Geometry: final body of the model. Coordinates: model frame, mm. A direction names the side the tool comes from. Round coordinates to 2 decimals unless told otherwise and drop trailing zeros. Loops run counter-clockwise (first coordinate to the right, second up) from the corner with the lowest first, then second, coordinate; pieces in that order, holes last. Notation, with made-up numbers: M 86,-30 L 139,-30 A9 cw 139,-18 Z; hole C 62,-4 d10. An arc over 180 degrees is marked long. Write each question's results on one line, items separated by ' | '.
```python
from build123d import *

# Parameters (mm, degrees)
BOSS_EXTRUDE1_DEPTH = 80
SKETCH2_W           = 20
SKETCH2_H           = 28
BOSS_EXTRUDE2_DEPTH = 10
FILLET1_R           = 7
CUT_EXTRUDE1_DEPTH  = 20
FILLET2_R           = 7
SKETCH4_R           = 3.2
CUT_EXTRUDE2_DEPTH  = 9.5


with BuildPart() as part:
    # Sketch1 → Boss-Extrude1 (new body)
    with BuildSketch(Plane.XY):
        Polygon((0, 0), (0, 34.685337878), (60.076767483, 0), align=None)
    extrude(amount=BOSS_EXTRUDE1_DEPTH)

    # Sketch2 → Boss-Extrude2 (add)
    with BuildSketch(Plane.XY.offset(80)):
        with Locations((10, -4)):
            Rectangle(SKETCH2_W, SKETCH2_H)
    boss_extrude2 = extrude(amount=BOSS_EXTRUDE2_DEPTH)

    # Fillet1
    fillet1_edges = [part.edges().sort_by_distance(p)[0] for p in [
        (20, 5, 80),
        (10, 10, 80),
    ]]
    fillet(fillet1_edges, radius=FILLET1_R)

    # Sketch3 → Cut-Extrude1 (cut)
    with BuildSketch(Plane.XY.offset(90)):
        with BuildLine():
            Line((7, -12), (7, -8))
            ThreePointArc((7, -8), (10, -5), (13, -8))
            Line((13, -8), (13, -12))
            ThreePointArc((13, -12), (10, -15), (7, -12))
        make_face()
    cut_extrude1 = extrude(amount=-CUT_EXTRUDE1_DEPTH, mode=Mode.SUBTRACT)

    # Mirror10: Boss-Extrude2, Cut-Extrude1 across plane
    add(boss_extrude2.mirror(Plane(origin=(0, 0, 40), x_dir=(1, 0, 0), z_dir=(0, 0, -1))))
    add(cut_extrude1.mirror(Plane(origin=(0, 0, 40), x_dir=(1, 0, 0), z_dir=(0, 0, -1))), mode=Mode.SUBTRACT)

    # Fillet2
    fillet2_edges = [part.edges().sort_by_distance(p)[0] for p in [
        (20, 5, 0),
        (10, 10, 0),
    ]]
    fillet(fillet2_edges, radius=FILLET2_R)

    # Sketch4 → Cut-Extrude2 (cut)
    with BuildSketch(Plane(origin=(15.019191871, 26.014003409, 0), x_dir=(0.8660254037844418, -0.49999999999999456, 0), z_dir=(0.4999999999999946, 0.8660254037844419, 0))):
        with Locations(Location((-6.342668939, -15, 0), (0, 0, 180))):
            Circle(SKETCH4_R)
        with Locations(Location((-6.342668939, -40, 0), (0, 0, 180))):
            Circle(SKETCH4_R)
        with Locations(Location((-6.342668939, -65, 0), (0, 0, 180))):
            Circle(SKETCH4_R)
    extrude(amount=-CUT_EXTRUDE2_DEPTH, mode=Mode.SUBTRACT)


solid = part.part
```
1. Pin query (flat end, axial travel): P1, Ø8, axis at x = 51.5, z = 27, coming from the +Y side; P2, Ø2.5, axis at x = 8, z = -8, coming from the +Y side; P3, Ø3, axis at y = -9.5, z = -2.5, coming from the +X side; P4, Ø6, axis at x = 38, y = 17.5, coming from the -Z side. Return the tip coordinate at first contact, or that it passes through.
Answer key:
P1: stops at y = 7.26 | P2: stops at y = 10 | P3: stops at x = 20 | P4: passes through
2. Access query for faces 5 (the face through (4.815, 20.936, 40.045)), 6 (the face through (13, -10, 85)), 7 (the face through (10, 10, 88)), 8 (the face through (20, -7, 85)). Directions: +Z, -Z, +X, -X, +Y, -Y. A direction counts if a zero-diameter tool reaches every point of the face in a straight line with its end or side. Return the directions, or none.
Answer key:
face 5: none | face 6: +Z, -Z | face 7: +Z, +X, -X, +Y | face 8: +Z, +X, -Y
3. Section A-A (y = -10). Output: boundary loops of the cut face in (x, z), then the cut area to 3 significant figures.
Answer key:
outline: M 0,-10 L 7,-10 L 7,0 L 0,0 Z; M 0,80 L 7,80 L 7,90 L 0,90 Z; M 13,-10 L 20,-10 L 20,0 L 13,0 Z; M 13,80 L 20,80 L 20,90 L 13,90 Z | area: 280 mm²
4. Draft query along X for faces 1 (the face through (30, 0, 39)), 2 (the face through (20, -7, -5)), 3 (the face through (7, -10, -5)), 4 (the face through (10, -15, 85)). Return one class per face: pulls with the +X half, pulls with the -X half, needs draft (parallel to the pull), parting line crosses it, or undercut.
Answer key:
face 1: needs draft | face 2: pulls with the +X half | face 3: undercut | face 4: undercut
5. Section B-B (x = 10). Count the separate pieces of the cut face and the enclosed holes in it, then the cut area to 3 significant figures.
Answer key:
separate pieces: 3 | enclosed holes: 0 | area: 2,620 mm²
6. Section C-C (z = 75). Output: boundary loops of the cut face in (x, y).
Answer key:
outline: M 0,0 L 60.08,0 L 0,34.69 Z
7. Ray query, probe 1 along Z at (x, y) = (19, -8); probe 2 along Z at (x, y) = (42.5, 9.5); probe 3 along Y at (x, z) = (21, 50). Return the intervals inside material, ascending.
Answer key:
probe 1: z = -10 to 0, 80 to 90 | probe 2: z = 0 to 80 | probe 3: y = 0 to 22.56
8. Section D-D (x = 32). Output: boundary loops of the cut face in (y, z), then the cut area to 3 significant figures.
Answer key:
outline: M 0,0 L 16.21,0 L 16.21,80 L 0,80 Z | area: 1,300 mm²
